```python
from build123d import *

# Parameters (mm, degrees)
SKIZZE1_W                       = 412.5
SKIZZE1_H                       = 412.5
AUFSATZ_LINEAR_AUSTRAGEN1_DEPTH = 15
SKIZZE2_W                       = 394.56
SKIZZE2_H                       = 394.56
SCHNITT_LINEAR_AUSTRAGEN1_DEPTH = 2
AUFSATZ_LINEAR_START            = -256.25
AUFSATZ_LINEAR_AUSTRAGEN2_DEPTH = 100


with BuildPart() as part:
    # Skizze1 → Aufsatz-Linear austragen1 (new body)
    with BuildSketch(Plane.XY):
        with Locations((206.25, -206.25)):
            Rectangle(SKIZZE1_W, SKIZZE1_H)
    extrude(amount=AUFSATZ_LINEAR_AUSTRAGEN1_DEPTH)

    # Skizze2 → Schnitt-Linear austragen1 (cut)
    with BuildSketch(Plane.XY.offset(15)):
        with Locations((206.25, -206.25)):
            Rectangle(SKIZZE2_W, SKIZZE2_H)
    extrude(amount=-SCHNITT_LINEAR_AUSTRAGEN1_DEPTH, mode=Mode.SUBTRACT)

    # Skizze3 → Aufsatz-Linear austragen2 (add)
    with BuildSketch(Plane(origin=(412.5, 0, 0), x_dir=(0, 0, -1), z_dir=(1, 0, 0)).offset(AUFSATZ_LINEAR_START)):
        Polygon((0, -206.25), (146.291749205, -360.735735275), (125.739095453, -368.119079257), (0, -235.337177889), align=None)
    extrude(amount=AUFSATZ_LINEAR_AUSTRAGEN2_DEPTH)


solid = part.part
```
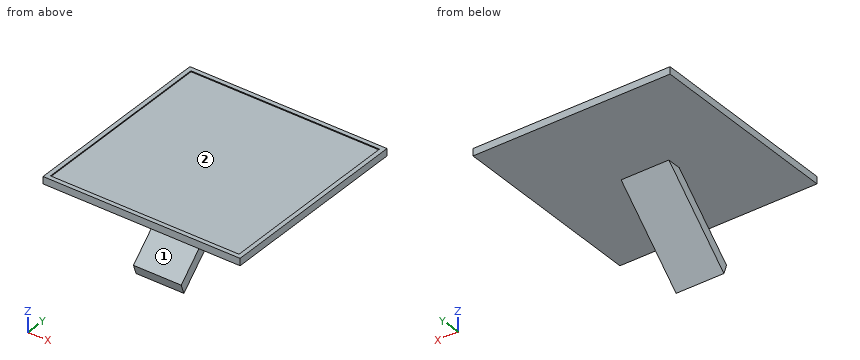
Here's how the part is built. I have some questions about the finished solid (model axes, mm). Face numbers are marked on the shaded views. Coordinates: 2 decimals unless noted, no trailing zeros. Write each loop counter-clockwise with the first axis right and the second up, starting at its lowest first coordinate (ties: lowest second). Pieces come first, ordered by that corner, then holes. Notation, with made-up numbers: (-8, 87) - (38, 87) arc R10 ccw to (38, 95) - close; hole circle Ø8 at (3, 54). An arc over 180 degrees is marked (long way). One line per item, written item: value.
1) I need wall thicknesses on line 1 along Z through (x, y) = (209, -172); line 2 along Y through (x, z) = (201, -60.5); line 3 along Y through (x, z) = (219, -108.5). Which ranges of each line are inside material? Lowest first, please.
Model answer:
line 1: z = 0 to 13
line 2: y = -299.23 to -270.14
line 3: y = -349.91 to -320.83
2) I'm going to push a flat-ended pin straight in: P1, Ø2, axis at x = 231.5, y = -226.5, coming from the +Z side. Where does the tip first touch, or does it pass through?
Model answer:
P1: stops at z = 13
3) Suppose I cut it at B-B on y = -173. Write out the boundary of the cut face in (x, z).
Model answer:
outline: (0, 0) - (412.5, 0) - (412.5, 15) - (403.53, 15) - (403.53, 13) - (8.97, 13) - (8.97, 15) - (0, 15) - close
4) Suppose I cut it at D-D on z = -45. Write out the boundary of the cut face in (x, y), and give its area (3 significant figures).
Model answer:
outline: (156.25, -282.86) - (256.25, -282.86) - (256.25, -253.77) - (156.25, -253.77) - close
area: 2,910 mm²
5) Suppose I cut it at C-C on y = -335.5. Write out the boundary of the cut face in (x, z), and give its area (3 significant figures).
Model answer:
outline: (0, 0) - (412.5, 0) - (412.5, 15) - (403.53, 15) - (403.53, 13) - (8.97, 13) - (8.97, 15) - (0, 15) - close; (156.25, -122.39) - (256.25, -122.39) - (256.25, -94.85) - (156.25, -94.85) - close
area: 8,150 mm²
6) Suppose I cut it at A-A on x = 271.5. Write out the boundary of the cut face in (y, z), and give its area (3 significant figures).
Model answer:
outline: (-412.5, 0) - (0, 0) - (0, 15) - (-8.97, 15) - (-8.97, 13) - (-403.53, 13) - (-403.53, 15) - (-412.5, 15) - close
area: 5,400 mm²
7) We'd pull the mould along X, two halves only. Please class the marked faces 1 and 2: pulls with the +X half, pulls with the -X half, needs draft (parallel to the pull), parting line crosses it, or undercut.
Model answer:
face 1: needs draft
face 2: undercut
